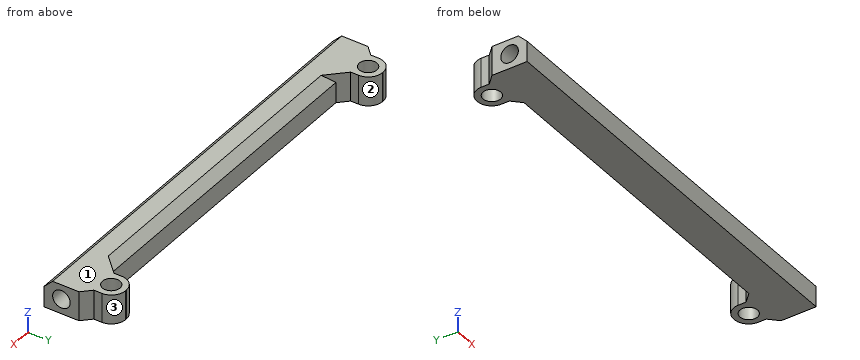
from build123d import *

# Parameters (mm, degrees)
SKETCH_W        = 72
SKETCH_H        = 6
PAD_DEPTH       = 2.5
SKETCH001_R     = 1.5
POCKET_DEPTH    = 11
SKETCH002_R     = 1.5
POCKET001_DEPTH = 11
SKETCH003_W     = 5
SKETCH003_H     = 5.85
SKETCH003_R     = 1.5
PAD001_DEPTH    = 5
CHAMFER_SIZE    = 1.49
FILLET_R        = 2.4
CHAMFER001_SIZE = 1.5


with BuildPart() as part:
    # Sketch → Pad (new body, symmetric)
    with BuildSketch(Plane.XY):
        Rectangle(SKETCH_W, SKETCH_H)
    extrude(amount=PAD_DEPTH, both=True)

    # Sketch001 → Pocket (cut)
    with BuildSketch(Plane(origin=(-36, 0, 0), x_dir=(0, -1, 0), z_dir=(-1, 0, 0))):
        Circle(SKETCH001_R)
    extrude(amount=-POCKET_DEPTH, mode=Mode.SUBTRACT)

    # Sketch002 → Pocket001 (cut)
    with BuildSketch(Plane.YZ.offset(36)):
        Circle(SKETCH002_R)
    extrude(amount=-POCKET001_DEPTH, mode=Mode.SUBTRACT)

    # Sketch003 → Pad001 (new body)
    with BuildSketch(Plane(origin=(0, 0, -2.5), x_dir=(1, 0, 0), z_dir=(0, 0, -1))):
        with Locations((32, -5.325)):
            Rectangle(SKETCH003_W, SKETCH003_H)
        with Locations((32, -5.75)):
            Circle(SKETCH003_R, mode=Mode.SUBTRACT)
        with Locations((-32, -5.325)):
            Rectangle(SKETCH003_W, SKETCH003_H)
        with Locations((-32, -5.75)):
            Circle(SKETCH003_R, mode=Mode.SUBTRACT)
    extrude(amount=-PAD001_DEPTH)

    # Chamfer
    chamfer_edges = [part.edges().sort_by_distance(p)[0] for p in [
        (34.5, 3, 0),
        (29.5, 3, 0),
        (-29.5, 3, 0),
        (-34.5, 3, 0),
    ]]
    chamfer(chamfer_edges, length=CHAMFER_SIZE)

    # Fillet
    fillet_edges = [part.edges().sort_by_distance(p)[0] for p in [
        (34.5, 8.25, 0),
        (29.5, 8.25, 0),
        (-29.5, 8.25, 0),
        (-34.5, 8.25, 0),
    ]]
    fillet(fillet_edges, radius=FILLET_R)

    # Chamfer001
    chamfer001_edges = [part.edges().sort_by_distance(p)[0] for p in [
        (0, -3, 2.5),
        (0, 3, 2.5),
    ]]
    chamfer(chamfer001_edges, length=CHAMFER001_SIZE)


solid = part.part
Source: CAD feature listing. Evaluate the final solid. Frame: model axes, mm. Face numbers are marked on the shaded views. Coordinates: 2 decimals unless noted, no trailing zeros. Order: outer loops, then holes, each group sorted by start corner. A loop starts at its lowest first (then second) coordinate and runs counter-clockwise, first axis right, second up. Notation, with made-up numbers: M 82.5,50.25 L 100.5,50.25 A16 ccw 100.5,63.25 Z; hole C 42.5,58 d7. An arc over 180 degrees is marked long. Write each question's results on one line, items separated by ' | '. Start each with the question number.
Item 1: First-contact query: pin 1 Ø4 at (x, y) = (5.5, 4) entering from +Z; pin 2 Ø2 at (x, z) = (14, -1.5) entering from +Y; pin 3 Ø0.9 at (y, z) = (0, -0.5) entering from +X; pin 4 Ø2.5 at (x, y) = (-32, 5.75) entering from -Z. Flat tips, straight axial feed; report the tip coordinate or a pass-through.
Item 2: Cut plane D-D (x = -8). Return loops of the section in (y, z).
Item 3: Cut plane B-B (z = 0). Count the separate pieces of the cut face and the enclosed holes in it, and give its area (3 significant figures).
Item 4: Line query: probe 1 along X at (y, z) = (5.75, -0.8); probe 2 along X at (y, z) = (7, 0.45); probe 3 along Y at (x, z) = (32, 0.25). Output: solid intervals per line, ascending.
Item 5: Draft query along X for the marked faces 1, 2 and 3. Return one class per face: pulls with the +X half, pulls with the -X half, needs draft (parallel to the pull), parting line crosses it, or undercut.
Item 6: Cut plane A-A (y = 6.5). Return loops of the section in (x, z), and give its area (3 significant figures).
Item 7: Cut plane C-C (y = 0). Return loops of the section in (x, z).
Checked values:
1) pin 1: stops at z = 2 | pin 2: stops at y = 3 | pin 3: stops at x = 25 | pin 4: passes through
2) outline: M -3,-2.5 L 3,-2.5 L 3,1 L 1.5,2.5 L -1.5,2.5 L -3,1 Z
3) separate pieces: 1 | enclosed holes: 2 | area: 404 mm2
4) probe 1: x = -34.5 to -33.5, -30.5 to -29.5, 29.5 to 30.5, 33.5 to 34.5 | probe 2: x = -34.21 to -32.83, -31.17 to -29.79, 29.79 to 31.17, 32.83 to 34.21 | probe 3: y = -3 to -1.48, 1.48 to 4.25, 7.25 to 8.25
5) face 1: needs draft | face 2: undercut | face 3: pulls with the +X half
6) outline: M -34.41,-2.5 L -33.3,-2.5 L -33.3,2.5 L -34.41,2.5 Z; M -30.7,-2.5 L -29.59,-2.5 L -29.59,2.5 L -30.7,2.5 Z; M 29.59,-2.5 L 30.7,-2.5 L 30.7,2.5 L 29.59,2.5 Z; M 33.3,-2.5 L 34.41,-2.5 L 34.41,2.5 L 33.3,2.5 Z | area: 22.2 mm2
7) outline: M -36,-2.5 L 36,-2.5 L 36,-1.5 L 25,-1.5 L 25,1.5 L 36,1.5 L 36,2.5 L -36,2.5 L -36,1.5 L -25,1.5 L -25,-1.5 L -36,-1.5 Z
